Drawing for the job (mm, zero at the part's lowest x, y, z). Coordinates: 2 decimals unless noted, no trailing zeros. Write each loop counter-clockwise with the first axis right and the second up, starting at its lowest first coordinate (ties: lowest second). Pieces come first, ordered by that corner, then holes.
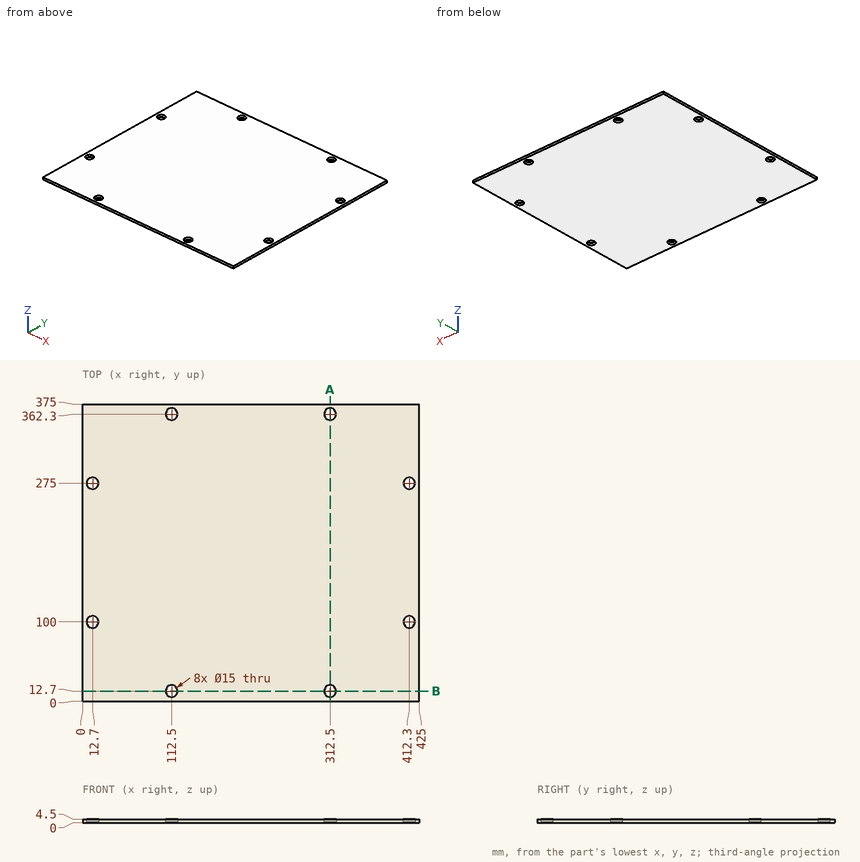
Item 1: Flat gauge pin, fed straight in: pin 1 Ø12 at (x, y) = (112.5, 362.3) entering from +Z. Where does the tip first touch, or does it go through?
Item 2: Saw through at B-B, the plane y = 12.7. Write the cut outline in (x, z), and give its area (3 significant figures).
Item 3: Wall check: line 1 along Y through (x, z) = (12.7, 3.55); line 2 along Y through (x, z) = (112.5, 3.35); line 3 along X through (y, z) = (105, 0.8). Give the ranges that are in metal, low to high.
Item 4: Saw through at A-A, the plane x = 312.5. Write the cut outline in (y, z).
Working result:
1. pin 1: passes through
2. outline: (0, 0) - (105, 0) - (105, 4.5) - (0, 4.5) - close; (120, 0) - (305, 0) - (305, 4.5) - (120, 4.5) - close; (320, 0) - (425, 0) - (425, 4.5) - (320, 4.5) - close
2. area: 1,780 mm2
3. line 1: y = 0 to 92.5, 107.5 to 267.5, 282.5 to 375
3. line 2: y = 0 to 5.2, 20.2 to 354.8, 369.8 to 375
3. line 3: x = 0 to 7.11, 18.29 to 406.71, 417.89 to 425
4. outline: (0, 0) - (5.2, 0) - (5.2, 4.5) - (0, 4.5) - close; (20.2, 0) - (354.8, 0) - (354.8, 4.5) - (20.2, 4.5) - close; (369.8, 0) - (375, 0) - (375, 4.5) - (369.8, 4.5) - close
